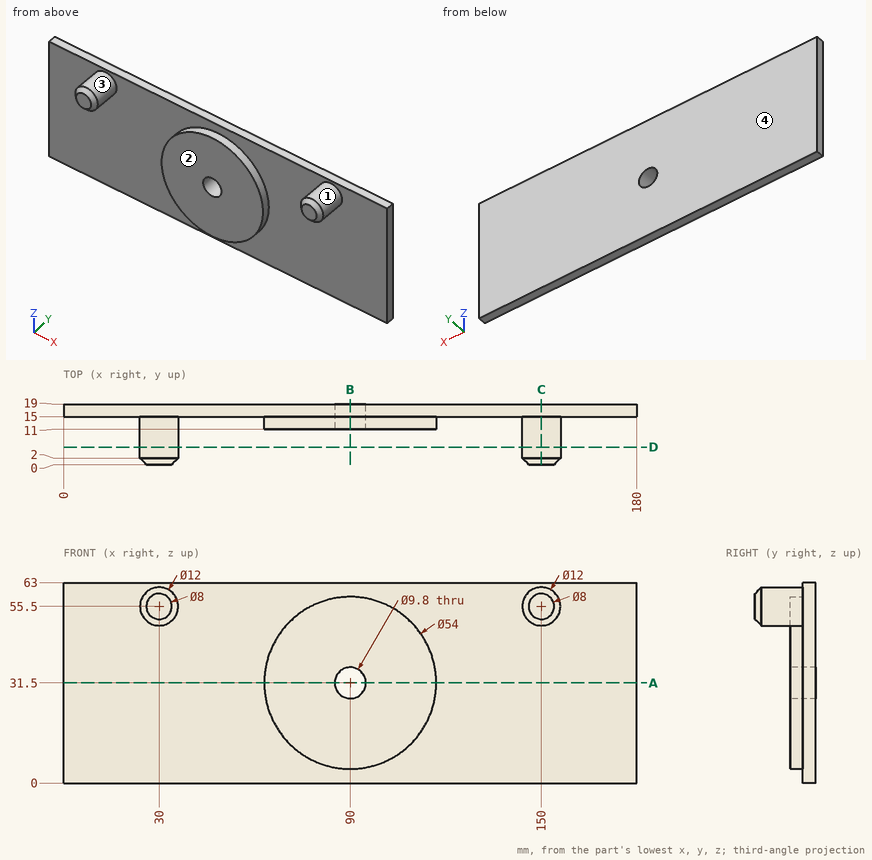
Study the drawing (mm; zero at the part's minimum x, y, z) and answer. A direction names the side the tool comes from. Round coordinates to 2 decimals unless told otherwise and drop trailing zeros. Loops run counter-clockwise (first coordinate to the right, second up) from the corner with the lowest first, then second, coordinate; pieces in that order, holes last. Notation, with made-up numbers: M 46,42.25 L 50,42.25 A13 ccw 50,66.25 Z; hole C 27.25,-0.75 d1. An arc over 180 degrees is marked long. One line per question, with ' | ' between items.
Q1. Consider line 1 along Z through (x, y) = (90, 14.25); line 2 along Z through (x, y) = (90, 16.5); line 3 along X through (y, z) = (12.5, 34.5). Determine where each line is inside the solid, lowest interval first. Write a range as from..to.
Conclusion:
line 1: z = 4.5..26.6, 36.4..58.5 | line 2: z = 0..26.6, 36.4..63 | line 3: x = 63.17..86.13, 93.87..116.83
Q2. Find section A-A, the plane z = 31.5. Give the vertices of the cut face in (x, y).
Conclusion:
outline: M 0,15 L 63,15 L 63,11 L 85.1,11 L 85.1,19 L 0,19 Z; M 94.9,11 L 117,11 L 117,15 L 180,15 L 180,19 L 94.9,19 Z
Q3. Find section D-D, the plane y = 5.5. Give the vertices of the cut face in (x, z), then the cut area to 3 significant figures.
Conclusion:
outline: C 30,55.5 d12; C 150,55.5 d12 | area: 226 mm2
Q4. The mould has two halves that part along X. Classify the marked faces 3 and 4: +X half, -X half, draft (parallel to the pull), parting line (faces both ways), or undercut.
Conclusion:
face 3: undercut | face 4: draft
Q5. Find section B-B, the plane x = 90. Give the vertices of the cut face in (y, z).
Conclusion:
outline: M 11,4.5 L 15,4.5 L 15,0 L 19,0 L 19,26.6 L 11,26.6 Z; M 11,36.4 L 19,36.4 L 19,63 L 15,63 L 15,58.5 L 11,58.5 Z
Q6. Find section C-C, the plane x = 150. Give the vertices of the cut face in (y, z), then the cut area to 3 significant figures.
Conclusion:
outline: M 0,51.5 L 2,49.5 L 15,49.5 L 15,0 L 19,0 L 19,63 L 15,63 L 15,61.5 L 2,61.5 L 0,59.5 Z | area: 428 mm2
Q7. A tool of negligible diameter and unlimited length cuts with its end or side. For the marked faces 1 and 2, from which of +Z, -Z, +X, -X, +Y, -Y can it reach the whole face along a straight path? Write none if from no direction.
Conclusion:
face 1: -Y | face 2: +Z, -Z, -Y
Q8. Each of these flat-tipped pins is pushed along its axis until it touches: pin 1 Ø16 at (x, z) = (86, 35) entering from -Y; pin 2 Ø1 at (x, y) = (154.5, 12) entering from +Z; pin 3 Ø3 at (y, z) = (12, 11) entering from +X. Where does it stop, or does it pass through?
Conclusion:
pin 1: stops at y = 11 | pin 2: stops at z = 59.97 | pin 3: stops at x = 109.18
